Verification items for the finished model (mm, model axes). Coordinates: 2 decimals unless noted, no trailing zeros. Write each loop counter-clockwise with the first axis right and the second up, starting at its lowest first coordinate (ties: lowest second). Pieces come first, ordered by that corner, then holes. Notation, with made-up numbers: (-25, -13) -> (22, -13) arc R24 ccw to (22, 9) -> close; hole circle Ø4 at (21, -35). An arc over 180 degrees is marked (long way). Answer in a Markdown table with one row per item.
```python
from build123d import *

# Parameters (mm, degrees)
SKETCH1_R           = 1.6
SKETCH1_R_2         = 6
BOSS_EXTRUDE1_DEPTH = 2
FILLET1_R           = 7


with BuildPart() as part:
    # Sketch1 → Boss-Extrude1 (new body)
    with BuildSketch(Plane(origin=(0, 0, 0), x_dir=(1, 0, 0), z_dir=(0, 1, 0))):
        Polygon((26, 0), (-13, 22.516660498), (-13, -22.516660498), align=None)
        with Locations((-7.5, 12.990381057)):
            Circle(SKETCH1_R, mode=Mode.SUBTRACT)
        with Locations((15, 0)):
            Circle(SKETCH1_R, mode=Mode.SUBTRACT)
        with Locations((-7.5, -12.990381057)):
            Circle(SKETCH1_R, mode=Mode.SUBTRACT)
        Circle(SKETCH1_R_2, mode=Mode.SUBTRACT)
    extrude(amount=BOSS_EXTRUDE1_DEPTH)

    # Fillet1
    fillet1_edges = [part.edges().sort_by_distance(p)[0] for p in [
        (-13, 1, 22.516660498),
        (-13, 1, -22.516660498),
        (26, 1, 0),
    ]]
    fillet(fillet1_edges, radius=FILLET1_R)


solid = part.part
```
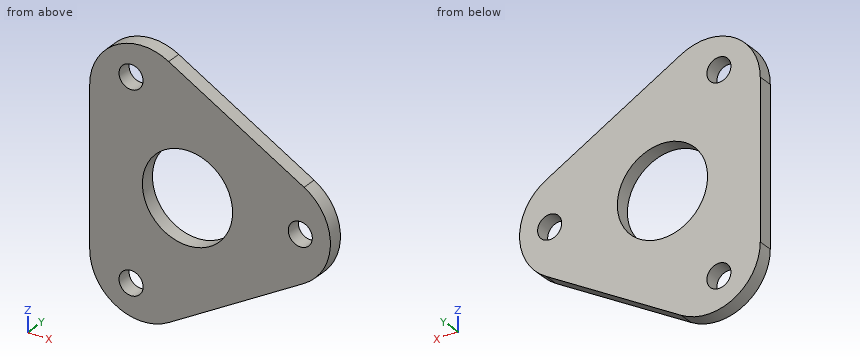
1. Section check C-C, the plane z = -4.5. Record the boundary of the cut face in (x, y).
Geometry says:
| item | result |
|---|---|
| outline | (-13, 0) -> (-3.97, 0) -> (-3.97, 2) -> (-13, 2) -> close; (3.97, 0) -> (17.36, 0) -> (17.36, 2) -> (3.97, 2) -> close |
2. Depth check by flat-ended pin: P1, Ø2.5, axis at x = -7.5, z = 12.99, coming from the +Y side. Enter the tip coordinate at first touch or a pass-through.
Geometry says:
| item | result |
|---|---|
| P1 | through |
3. Section check A-A, the plane z = 0. Record the boundary of the cut face in (x, y), plus the area to 3 significant figures.
Geometry says:
| item | result |
|---|---|
| outline | (-13, 0) -> (-6, 0) -> (-6, 2) -> (-13, 2) -> close; (6, 0) -> (13.4, 0) -> (13.4, 2) -> (6, 2) -> close; (16.6, 0) -> (19, 0) -> (19, 2) -> (16.6, 2) -> close |
| area | 33.6 mm^2 |
4. Section check D-D, the plane y = 1.1. Record the boundary of the cut face in (x, z).
Geometry says:
| item | result |
|---|---|
| outline | (-13, -10.39) arc R7 ccw to (-2.5, -16.45) -> (15.5, -6.06) arc R7 ccw to (15.5, 6.06) -> (-2.5, 16.45) arc R7 ccw to (-13, 10.39) -> close; hole circle Ø3.2 at (-7.5, -12.99); hole circle Ø3.2 at (-7.5, 12.99); hole circle Ø12 at (0, 0); hole circle Ø3.2 at (15, 0) |
5. Section check B-B, the plane x = -7.5. Record the boundary of the cut face in (y, z).
Geometry says:
| item | result |
|---|---|
| outline | (0, -17.23) -> (2, -17.23) -> (2, -14.59) -> (0, -14.59) -> close; (0, -11.39) -> (2, -11.39) -> (2, 11.39) -> (0, 11.39) -> close; (0, 14.59) -> (2, 14.59) -> (2, 17.23) -> (0, 17.23) -> close |
6. Thickness scan on line 1 (X direction, y = 1.3, z = 0); line 2 (Z direction, x = -7.5, y = 0.6); line 3 (X direction, y = 0.55, z = 5). Record the ranges inside material, lowest first. Write a range as from..to.
Geometry says:
| item | result |
|---|---|
| line 1 | -13..-6, 6..13.4, 16.6..19 |
| line 2 | -17.23..-14.59, -11.39..11.39, 14.59..17.23 |
| line 3 | -13..-3.32, 3.32..16.9 |
